Work out the finished part from the listing and answer in its coordinate system (mm). Give positions to 0.01 mm unless a question says otherwise; leave off trailing zeros. Write each loop counter-clockwise with the first axis right and the second up, starting at its lowest first coordinate (ties: lowest second). Pieces come first, ordered by that corner, then holes. Notation, with made-up numbers: (-35.5, 7.5) -> (21.5, 7.5) arc R27 cw to (21.5, 34.5) -> close; hole circle Ø4 at (-4, 16). An arc over 180 degrees is marked (long way). Use a Markdown table: item, result. Add a question column.
Q1. Section A-A, the plane y = 1.25 is taken. Give the vertices of the cut face in (x, z), plus the area to 3 significant figures.
Q2. Each of these flat-tipped pins is pushed along its axis until it touches: pin 1 Ø1 at (y, z) = (1.5, 2) entering from -X; pin 2 Ø1 at (x, z) = (-253.5, -26.5) entering from -Y; pin 3 Ø1.6 at (x, y) = (-22, 1) entering from -Z. Where does it stop, or does it pass through?
Q3. Consider line 1 (X direction, y = 0.25, z = -51); line 2 (Z direction, x = -39, y = 1.95). Determine where each line is inside the solid, lowest interval first.
Q4. Section B-B, the plane x = -40 is taken. Give the vertices of the cut face in (y, z) (3 decimals).
from build123d import *

# Parameters (mm, degrees)
SKETCH1_W           = 287.02
SKETCH1_H           = 50.8
BOSS_EXTRUDE1_DEPTH = 3.175
SKETCH2_W           = 175.006
SKETCH2_H           = 5.9436
BOSS_EXTRUDE2_DEPTH = 3.175
FILLET1_R           = 2.54
FILLET2_R           = 2.54


with BuildPart() as part:
    # Sketch1 → Boss-Extrude1 (new body)
    with BuildSketch(Plane(origin=(0, 0, 0), x_dir=(1, 0, 0), z_dir=(0, 1, 0))):
        with Locations((-143.51, 25.4)):
            Rectangle(SKETCH1_W, SKETCH1_H)
    extrude(amount=BOSS_EXTRUDE1_DEPTH)

    # Sketch2 → Boss-Extrude2 (add)
    with BuildSketch(Plane(origin=(0, 3.175, 0), x_dir=(1, 0, 0), z_dir=(0, 1, 0))):
        with Locations((-142.367, -2.9718)):
            Rectangle(SKETCH2_W, SKETCH2_H)
        with Locations((-142.367, 53.7718)):
            Rectangle(SKETCH2_W, SKETCH2_H)
    extrude(amount=-BOSS_EXTRUDE2_DEPTH)

    # Fillet1
    fillet1_edges = [part.edges().sort_by_distance(p)[0] for p in [
        (0, 1.5875, -50.8),
        (0, 1.5875, 0),
    ]]
    fillet(fillet1_edges, radius=FILLET1_R)

    # Fillet2
    fillet2_edges = [part.edges().sort_by_distance(p)[0] for p in [
        (-287.02, 1.5875, 0),
        (-287.02, 1.5875, -50.8),
    ]]
    fillet(fillet2_edges, radius=FILLET2_R)


solid = part.part
Result set:
| question | item | result |
|---|---|---|
| 1 | outline | (-287.02, -48.26) arc R2.54 ccw to (-284.48, -50.8) -> (-229.87, -50.8) -> (-229.87, -56.74) -> (-54.86, -56.74) -> (-54.86, -50.8) -> (-2.54, -50.8) arc R2.54 ccw to (0, -48.26) -> (0, -2.54) arc R2.54 ccw to (-2.54, 0) -> (-54.86, 0) -> (-54.86, 5.94) -> (-229.87, 5.94) -> (-229.87, 0) -> (-284.48, 0) arc R2.54 ccw to (-287.02, -2.54) -> close |
| 1 | area | 16,700 mm2 |
| 2 | pin 1 | stops at x = -229.87 |
| 2 | pin 2 | stops at y = 0 |
| 2 | pin 3 | stops at z = -50.8 |
| 3 | line 1 | x = -229.87 to -54.86 |
| 3 | line 2 | z = -50.8 to 0 |
| 4 | outline | (0, -50.8) -> (3.175, -50.8) -> (3.175, 0) -> (0, 0) -> close |
